Here's how the part is built. I have some questions about the finished solid (model axes, mm). Face numbers are marked on the shaded views. A direction names the side the tool comes from. Round coordinates to 2 decimals unless told otherwise and drop trailing zeros. Loops run counter-clockwise (first coordinate to the right, second up) from the corner with the lowest first, then second, coordinate; pieces in that order, holes last. Notation, with made-up numbers: M 76,-10.75 L 99,-10.75 A15 ccw 99,-2.75 Z; hole C 31,50 d10. An arc over 180 degrees is marked long. Answer as a JSON object with one key per item and string values.
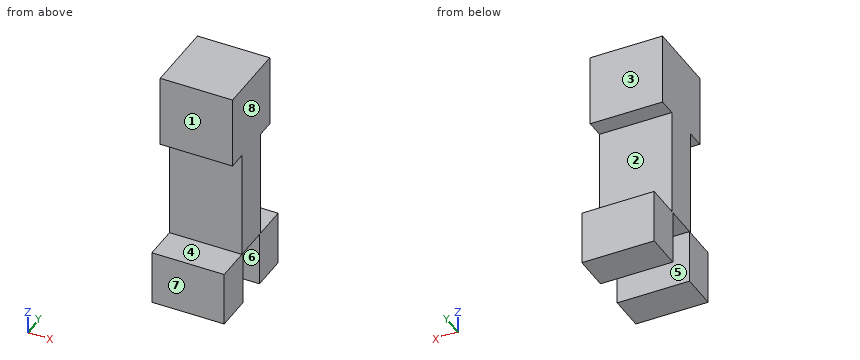
from build123d import *

# Parameters (mm, degrees)
F0_W     = 80
F0_H     = 80
F1_DEPTH = 80
F2_W     = 80
F2_H     = 40
F3_DEPTH = 120
F4_W     = 80
F4_H     = 40
F5_DEPTH = 60


with BuildPart() as f1:
    # F0 (on Top) → F1 (new body)
    with BuildSketch(Plane.XY):
        with Locations((-17.931859, 10.016291)):
            Rectangle(F0_W, F0_H)
    extrude(amount=F1_DEPTH)

    # F2 (on face) → F3 (join)
    with BuildSketch(Plane(origin=(0, 0, 0), x_dir=(1, 0, 0), z_dir=(0, 0, -1))):
        with Locations((-17.931859, -10.016291)):
            Rectangle(F2_W, F2_H)
    extrude(amount=F3_DEPTH)

    # F4 (on face) → F5 (join)
    with BuildSketch(Plane(origin=(0, 0, -120), x_dir=(1, 0, 0), z_dir=(0, 0, -1))):
        with Locations((-17.931859, 27.983709)):
            Rectangle(F4_W, F4_H)
        with Locations((-17.931859, -48.016291)):
            Rectangle(F4_W, F4_H)
    extrude(amount=F5_DEPTH)


solid = f1.part
Item 1: On a 3-axis mill with a long thin cutter (end or side, diameter ignored), from which of +Z, -Z, +X, -X, +Y, -Y can I reach the whole of each face in a straight line? I mean the marked faces 1, 2, 3 and 4. Say none if no direction works.
Resolved:
{"face 1": "+Z, +X, -X, -Y", "face 2": "+X, -X, +Y", "face 3": "+Z, +X, -X, +Y", "face 4": "+X, -X, -Y"}
Item 2: I want a section at D-D, the plane z = -16.5. Please give me the cut outline in (x, y).
Resolved:
{"outline": "M -57.93,-9.98 L 22.07,-9.98 L 22.07,30.02 L -57.93,30.02 Z"}
Item 3: I'm going to push flat-ended pins straight in: pin 1 Ø6 at (x, z) = (-49.5, -62) entering from -Y; pin 2 Ø10 at (x, z) = (2, 51.5) entering from -Y; pin 3 Ø1 at (x, z) = (-29, -46) entering from +Y. Where does each tip first touch, or does it pass through?
Resolved:
{"pin 1": "y = -9.98", "pin 2": "y = -29.98", "pin 3": "y = 30.02"}
Item 4: I want a section at C-C, the plane x = -16. Please give me the cut outline in (y, z).
Resolved:
{"outline": "M -47.98,-180 L -7.98,-180 L -7.98,-120 L 28.02,-120 L 28.02,-180 L 68.02,-180 L 68.02,-120 L 30.02,-120 L 30.02,0 L 50.02,0 L 50.02,80 L -29.98,80 L -29.98,0 L -9.98,0 L -9.98,-120 L -47.98,-120 Z"}
Item 5: I want a section at A-A, the plane y = -25. Please give me the cut outline in (x, z).
Resolved:
{"outline": "M -57.93,-180 L 22.07,-180 L 22.07,-120 L -57.93,-120 Z; M -57.93,0 L 22.07,0 L 22.07,80 L -57.93,80 Z"}
Item 6: Please list where these lines run through material, in increasing order: probe 1 along Y at (x, z) = (-29, -155.5); probe 2 along Z at (x, y) = (18, 48); probe 3 along Z at (x, y) = (-43.5, 2.5). Write a range as from..to.
Resolved:
{"probe 1": "-47.98..-7.98, 28.02..68.02", "probe 2": "-180..-120, 0..80", "probe 3": "-120..80"}
Item 7: If we mould it in two halves opening along Y, with no side actions, what happens to the marked faces 5, 6, 7 and 8? For each: pulls with the +Y half, pulls with the -Y half, needs draft (parallel to the pull), parting line crosses it, or undercut.
Resolved:
{"face 5": "undercut", "face 6": "undercut", "face 7": "pulls with the -Y half", "face 8": "needs draft"}
Item 8: I want a section at B-B, the plane z = -127. Please give me the cut outline in (x, y).
Resolved:
{"outline": "M -57.93,-47.98 L 22.07,-47.98 L 22.07,-7.98 L -57.93,-7.98 Z; M -57.93,28.02 L 22.07,28.02 L 22.07,68.02 L -57.93,68.02 Z"}
